Build history of the part. All positions in model axes, mm. Give positions to 0.01 mm unless a question says otherwise; leave off trailing zeros. Write item = value, one per line. Start each with the question number.
Q1. Wall check: line 1 (Y direction, x = 153, z = -2.2); line 2 (X direction, y = 48, z = -0.95); line 3 (X direction, y = 85, z = -1.3). Give the ranges that are in metal, low to high.
Q2. Saw through at A-A, the plane z = -0.6. Give the number of separate pieces and of enclosed holes in the cut face, then the cut area to 3 significant figures.
Q3. Drop flat-ended pins along their axis: P1, Ø1.5, axis at x = 204.5, z = -1, coming from the +Y side; P2, Ø2.5, axis at x = 153, y = 208, coming from the -Z side; P3, Ø4.5, axis at x = 53, y = -15, coming from the -Z side; P4, Ø1, axis at y = 106.5, z = -2, coming from the +X side. Give the stop position or say it passes through.
Autodesk Inventor part; units mm, degrees
ref_plane "YZ Plane" through (0, 0, 0) normal (1, 0, 0) x (0, 1, 0)
ref_plane "XZ Plane" through (0, 0, 0) normal (0, 1, 0) x (-1, 0, 0)
ref_plane "XY Plane" through (0, 0, 0) normal (0, 0, 1) x (1, 0, 0)
sketch "Boceto1" plane through (0, 0, 0) normal (0, 0, 1) x (1, 0, 0)
  line L0 (206, -30) -> (206, 220)
  line L1 (0, 220) -> (206, 220)
  line L2 (0, -30) -> (0, 220)
  line L3 (206, -30) -> (0, -30)
  line L4 (206, -30) -> (206, -5)
  line L5 (206, -5) -> (203, -5)
  line L6 (203, -5) -> (203, 20)
  line L7 (203, 20) -> (206, 20)
  line L8 (206, 20) -> (206, 45)
  line L9 (206, 45) -> (203, 45)
  line L10 (203, 45) -> (203, 70)
  line L11 (203, 70) -> (206, 70)
  line L12 (206, 70) -> (206, 95)
  line L13 (206, 95) -> (203, 95)
  line L14 (203, 95) -> (203, 120)
  line L15 (203, 120) -> (206, 120)
  line L16 (206, 120) -> (206, 145)
  line L17 (206, 145) -> (203, 145)
  line L18 (203, 145) -> (203, 170)
  line L19 (203, 170) -> (206, 170)
  line L20 (203, 220) -> (206, 220)
  line L21 (206, 195) -> (203, 195)
  line L22 (203, 195) -> (203, 220)
  line L23 (206, 170) -> (206, 195)
  line L24 (203, 170) -> (206, 170)
  line L25 (0, 220) -> (0, 195)
  line L26 (0, 195) -> (3, 195)
  line L27 (3, 195) -> (3, 170)
  line L28 (3, 170) -> (0, 170)
  line L29 (0, 170) -> (0, 145)
  line L30 (0, 145) -> (3, 145)
  line L31 (3, 145) -> (3, 120)
  line L32 (3, 120) -> (0, 120)
  line L33 (3, 20) -> (0, 20)
  line L34 (0, 45) -> (3, 45)
  line L35 (3, 45) -> (3, 20)
  line L36 (0, 70) -> (0, 45)
  line L37 (3, 70) -> (0, 70)
  line L38 (3, 95) -> (3, 70)
  line L39 (0, 95) -> (3, 95)
  line L40 (0, 120) -> (0, 95)
  line L41 (3, 20) -> (0, 20)
  line L42 (0, 20) -> (0, -5)
  line L43 (0, -5) -> (3, -5)
  line L44 (3, -5) -> (3, -30)
  line L45 (3, -30) -> (0, -30)
  line L46 (203, 220) -> (206, 220)
  line L47 (203, 220) -> (206, 220)
  line L48 (206, 220) -> (206, 245)
  line L49 (206, 245) -> (203, 245)
  line L50 (203, 245) -> (203, 270)
  line L51 (203, 270) -> (206, 270)
  line L52 (0, 220) -> (3, 220)
  line L53 (0, 220) -> (3, 220)
  line L54 (3, 220) -> (3, 245)
  line L55 (3, 245) -> (0, 245)
  line L56 (0, 245) -> (0, 270)
  line L57 (0, 270) -> (3, 270)
  line L58 (206, 270) -> (0, 270)
  point P0 (0, 0)
  dimension "d78" = 3
  dimension "d88" = 3
  dimension "Lengueta" = 25
  dimension "espesor" = 3
  dimension "d2" = 25
  dimension "d3" = 3
  dimension "d4" = 25
  dimension "d5" = 90
  dimension "d6" = 3
  dimension "d7" = 25
  dimension "d8" = 3
  dimension "d9" = 25
  dimension "d10" = 3
  dimension "d11" = 25
  dimension "d12" = 3
  dimension "d13" = 25
  dimension "d14" = 90
  dimension "d15" = 3
  dimension "d16" = 25
  dimension "d17" = 3
  dimension "d18" = 3
  dimension "d19" = 25
  dimension "d20" = 90
  dimension "d21" = 3
  dimension "d22" = 25
  dimension "d23" = 3
  dimension "d26" = 25
  dimension "d27" = 3
  dimension "d28" = 25
  dimension "d29" = 3
  dimension "d30" = 25
  dimension "d31" = 90
  dimension "d32" = 3
  dimension "d33" = 25
  dimension "d34" = 3
  dimension "d35" = 25
  dimension "d36" = 3
  dimension "d37" = 25
  dimension "d38" = 3
  dimension "d39" = 25
  dimension "d40" = 90
  dimension "d41" = 3
  dimension "d42" = 25
  dimension "d43" = 3
  dimension "d44" = 3
  dimension "d45" = 25
  dimension "d46" = 90
  dimension "d47" = 3
  dimension "d48" = 25
  dimension "d49" = 3
  dimension "d71" = 3
  dimension "d72" = 3
  dimension "d73" = 25
  dimension "d74" = 90
  dimension "d75" = 3
  dimension "d76" = 25
  dimension "d77" = 3
  dimension "d81" = 3
  dimension "d82" = 3
  dimension "d83" = 25
  dimension "d84" = 90
  dimension "d85" = 3
  dimension "d86" = 25
  dimension "d87" = 3
extrude "Extrusión1" add sketch "Boceto1" against normal blind 3 contours L3 L44 L43 L2 L33 L35 L34 L37 L38 L39 L32 L31 L30 L28 L27 L26 L1 L22 L21 L0 L19 L18 L17 L15 L14 L13 L11 L10 L9 L7 L6 L5
sketch "Boceto2" plane through (0, 0, 0) normal (0, 0, 1) x (1, 0, 0)
  circle A0 centre (53, -15) radius 1.75
  circle A1 centre (153, -15) radius 1.75
  point P0 (0, 0)
extrude "Extrusión2" cut sketch "Boceto2" against normal blind 3
sketch "Boceto3" plane through (0, 0, 0) normal (0, 0, 1) x (1, 0, 0)
  circle A0 centre (53, 208) radius 2.1
  circle A1 centre (53, 208) radius 1.5
  circle A2 centre (153, 208) radius 2.1
  point P0 (0, 0)
  dimension "d56" = 3
hole "Agujero1" at (53, 208, 0) at (153, 208, 0) direction (0, 0, -1) diameter 3 depth 4
sketch "Boceto4" plane through (0, 0, 0) normal (0, 0, 1) x (1, 0, 0)
  circle A0 centre (53, 85) radius 2.1
  circle A1 centre (153, 85) radius 2.1
  point P0 (0, 0)
hole "Agujero2" at (153, 85, 0) at (53, 85, 0) direction (0, 0, -1) diameter 3 depth 4
sketch "Boceto5" plane through (0, 0, -3) normal (0, 0, -1) x (-1, 0, 0)
  point P0 (0, 0)
sketch "Boceto6" plane through (0, 0, 0) normal (0, 0, 1) x (1, 0, 0)
  circle A0 centre (53, 85) radius 1.5
  circle A1 centre (153, 85) radius 1.5
  circle A2 centre (153, 208) radius 1.5
  circle A3 centre (53, 208) radius 1.5
  circle A4 centre (53, -15) radius 1.75
  circle A5 centre (153, -15) radius 1.75
  line L0 (203, 20) -> (206, 20)
  line L1 (206, 20) -> (206, 45)
  line L2 (206, 45) -> (203, 45)
  line L3 (203, 45) -> (203, 70)
  line L4 (203, 70) -> (206, 70)
  line L5 (206, 70) -> (206, 95)
  line L6 (206, 95) -> (203, 95)
  line L7 (203, 95) -> (203, 120)
  line L8 (203, 120) -> (206, 120)
  line L9 (206, 120) -> (206, 145)
  line L10 (206, 145) -> (203, 145)
  line L11 (203, 145) -> (203, 170)
  line L12 (203, 170) -> (206, 170)
  line L13 (206, 170) -> (206, 195)
  line L14 (206, 195) -> (203, 195)
  line L15 (203, 195) -> (203, 220)
  line L16 (203, 220) -> (0, 220)
  line L17 (0, 220) -> (0, 195)
  line L18 (0, 195) -> (3, 195)
  line L19 (3, 195) -> (3, 170)
  line L20 (3, 170) -> (0, 170)
  line L21 (0, 170) -> (0, 145)
  line L22 (0, 145) -> (3, 145)
  line L23 (3, 145) -> (3, 120)
  line L24 (3, 120) -> (0, 120)
  line L25 (0, 120) -> (0, 95)
  line L26 (0, 95) -> (3, 95)
  line L27 (3, 95) -> (3, 70)
  line L28 (3, 70) -> (0, 70)
  line L29 (0, 70) -> (0, 45)
  line L30 (0, 45) -> (3, 45)
  line L31 (3, 45) -> (3, 20)
  line L32 (3, 20) -> (0, 20)
  line L33 (0, 20) -> (0, -5)
  line L34 (0, -5) -> (3, -5)
  line L35 (3, -5) -> (3, -30)
  line L36 (3, -30) -> (206, -30)
  line L37 (206, -30) -> (206, -5)
  line L38 (206, -5) -> (203, -5)
  line L39 (203, -5) -> (203, 20)
  line L40 (153, 85) -> (153, 208)
  line L41 (150.5, 161.5) -> (155.5, 161.5)
  line L42 (155.5, 161.5) -> (155.5, 131.5)
  line L43 (155.5, 131.5) -> (150.5, 131.5)
  line L44 (150.5, 131.5) -> (150.5, 161.5)
  line L45 (150.5, 161.5) -> (155.5, 131.5) construction
  line L46 (155.5, 161.5) -> (150.5, 131.5) construction
  line L47 (53, 85) -> (53, 208)
  line L48 (50.5, 161.5) -> (55.5, 161.5)
  line L49 (55.5, 161.5) -> (55.5, 131.5)
  line L50 (55.5, 131.5) -> (50.5, 131.5)
  line L51 (50.5, 131.5) -> (50.5, 161.5)
  line L52 (50.5, 161.5) -> (55.5, 131.5) construction
  line L53 (55.5, 161.5) -> (50.5, 131.5) construction
  line L54 (53, -15) -> (53, 85)
  line L55 (50.5, 50) -> (55.5, 50)
  line L56 (55.5, 50) -> (55.5, 20)
  line L57 (55.5, 20) -> (50.5, 20)
  line L58 (50.5, 20) -> (50.5, 50)
  line L59 (50.5, 50) -> (55.5, 20) construction
  line L60 (55.5, 50) -> (50.5, 20) construction
  line L61 (150.5, 50) -> (155.5, 50)
  line L62 (155.5, 50) -> (155.5, 20)
  line L63 (155.5, 20) -> (150.5, 20)
  line L64 (150.5, 20) -> (150.5, 50)
  line L65 (150.5, 50) -> (155.5, 20) construction
  line L66 (155.5, 50) -> (150.5, 20) construction
  point P0 (0, 0)
  point P1 (153, 146.5)
  point P2 (53, 146.5)
  point P3 (53, 35)
  point P4 (153, 35)
  dimension "d93" = 5
  dimension "d94" = 30
  dimension "d95" = 5
  dimension "d96" = 30
  dimension "d99" = 5
  dimension "d100" = 30
  dimension "d101" = 5
  dimension "d102" = 30
extrude "Extrusión3" cut sketch "Boceto6" against normal blind 3 contours L55 L56 L57 L54 | L54 L57 L58 L55 | L50 L51 L48 L47 | L47 L48 L49 L50 | L43 L44 L41 L40 | L40 L41 L42 L43 | L61 L62 L63 L64
sketch "Boceto7" plane through (0, 0, 0) normal (0, 0, 1) x (1, 0, 0)
  line L0 (203, 220) -> (0, 220)
  line L1 (0, 220) -> (3, 220)
  line L2 (3, 220) -> (10.5, 220)
  line L3 (10.5, 220) -> (10.5, 216.6)
  circle A0 centre (10.5, 218.3) radius 1.7
  line L4 (8.8, 218.3) -> (8.8, 220)
  line L5 (12.2, 218.3) -> (12.2, 220)
  point P0 (0, 0)
  dimension "d105" = 3
  dimension "d106" = 7.5
  dimension "d107" = 3.4
extrude "Extrusión4" cut sketch "Boceto7" against normal blind 10
equation "\"d2\" = Lengueta"
equation "\"d3\" = espesor"
equation "\"d4\" = Lengueta"
equation "\"d6\" = espesor"
equation "\"d7\" = Lengueta"
equation "\"d8\" = espesor"
equation "\"d11\" = d9"
equation "\"d12\" = d10"
equation "\"d13\" = d9"
equation "\"d16\" = d9"
equation "\"d18\" = d24"
equation "\"d19\" = d25"
equation "\"d22\" = d25"
equation "\"d28\" = d26"
equation "\"d29\" = d27"
equation "\"d30\" = d26"
equation "\"d33\" = d26"
equation "\"d37\" = d35"
equation "\"d38\" = d36"
equation "\"d39\" = d35"
equation "\"d42\" = d35"
equation "\"d44\" = d50"
equation "\"d45\" = d51"
equation "\"d48\" = d51"
equation "\"d71\" = d78"
equation "\"d72\" = d79"
equation "\"d73\" = d80"
equation "\"d76\" = d80"
equation "\"d81\" = d88"
equation "\"d82\" = d89"
equation "\"d83\" = d90"
equation "\"d86\" = d90"
equation "\"d52\" = espesor"
equation "\"d54\" = espesor"
properties part number "Envolvente_Pared_Derecha"
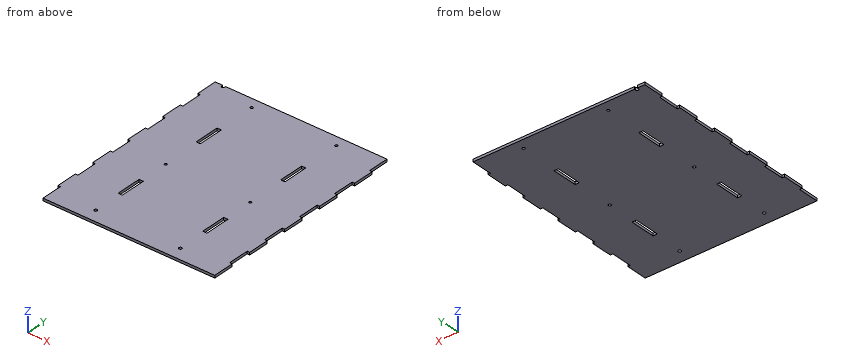
Report:
q1.line_1 = -30 to -16.75, -13.25 to 20, 50 to 83.5, 86.5 to 131.5, 161.5 to 206.5, 209.5 to 220
q1.line_2 = 0 to 50.5, 55.5 to 150.5, 155.5 to 203
q1.line_3 = 3 to 51.5, 54.5 to 151.5, 154.5 to 206
q2.separate_pieces = 1
q2.enclosed_holes = 10
q2.area = 50,100 mm2
q3.P1 = 195
q3.P2 = through
q3.P3 = -3
q3.P4 = 203
